For this review, take the finished solid that the model builds, in its own axes (mm). A direction names the side the tool comes from. Round coordinates to 2 decimals unless told otherwise and drop trailing zeros. Order: outer loops, then holes, each group sorted by start corner. A loop starts at its lowest first (then second) coordinate and runs counter-clockwise, first axis right, second up. Notation, with made-up numbers: (81, -17) -> (136, -17) arc R20 cw to (136, 10) -> close; hole circle Ø8 at (0, 13.25). An arc over 180 degrees is marked (long way). Use a Markdown table: item, result. Add a question column.
1) Machinability: for faces 4 (the face through (3, 54, -14)), 5 (the face through (-38.556, 93.156, -36.092)), 6 (the face through (-34.17, 64.54, -36.5)), 7 (the face through (-3, 54, -14)), which of the approach directions +Z, -Z, +X, -X, +Y, -Y give a long, thin tool a straight path to every point of the face, cutting with its end or side? Answer none if there is none.
2) Wall thickness on line 1 along Y through (x, z) = (-36, 27); line 2 along Y through (x, z) = (-32, 16.5); line 3 along Z through (x, y) = (17, 89.5): over which ranges is each line inside the solid? List them lowest first. Write a range as [from, to].
3) Consider section B-B (y = 23). State the section outline as (x, z) points.
4) Consider section A-A (y = 101.5). State the section outline as (x, z) points, plus the area to 3 significant figures.
5) Clearance check with flat-ended pins moving along their axes: P1, Ø3.5, axis at y = 54.5, z = -14, coming from the +X side; P2, Ø1.5, axis at y = 55.5, z = -11, coming from the -X side; P3, Ø12, axis at x = -7, z = -46.5, coming from the -Y side. State where each tip first meets the part, or that it passes through.
6) Consider section C-C (y = 9). State the section outline as (x, z) points.
7) Draft analysis for pull direction Y (two halves, no side actions). For faces 1 (the face through (-34, 109, -34)), 2 (the face through (-10, 0, -10)), 3 (the face through (-38.327, 95.965, -35.879)), state which applies: pulls with the +Y half, pulls with the -Y half, needs draft (parallel to the pull), parting line crosses it, or undercut.
Autodesk Fusion 360 part; units mm, degrees
sketch "Sketch1" plane through (0, 0, 0) normal (0, 0, 1) x (1, 0, 0)
  line L0 (12.5, 0) -> (22.5, 0)
  line L1 (12.5, 0) -> (12.5, 20)
  line L2 (22.5, 0) -> (22.5, 20)
  line L3 (22.5, 20) -> (42.5, 20)
  line L4 (42.5, 20) -> (42.5, 25)
  line L5 (42.5, 25) -> (22.5, 25)
  line L6 (0, 0) -> (0, 115)
  line L7 (0, 25) -> (0, 41)
  line L8 (22.5, 41) -> (47.5, 41)
  line L9 (47.5, 41) -> (47.5, 46)
  line L10 (47.5, 46) -> (22.5, 46)
  line L11 (0, 46) -> (0, 62)
  line L12 (22.5, 62) -> (50, 62)
  line L13 (50, 62) -> (50, 67)
  line L14 (50, 67) -> (22.5, 67)
  line L15 (0, 67) -> (0, 83)
  line L16 (57.5, 83) -> (57.5, 88)
  line L17 (0, 88) -> (0, 104)
  line L18 (65, 104) -> (65, 109)
  line L19 (52.5, 98.5) -> (52.5, 93.5)
  line L20 (65, 104) -> (52.5, 98.5)
  line L21 (52.5, 93.5) -> (57.5, 88)
  line L22 (12.5, 20) -> (12.5, 109)
  line L23 (22.5, 20) -> (22.5, 109)
  line L24 (0, 83) -> (0, 77.5)
  line L25 (23, 77.5) -> (42.5, 77.5)
  line L26 (42.5, 77.5) -> (42.5, 72.5)
  line L27 (42.5, 72.5) -> (22.5, 72.5041)
  line L28 (42.5, 77.5) -> (57.5, 83)
  line L29 (42.5, 72.5) -> (50, 67)
  line L30 (0, 62) -> (0, 56.5)
  line L31 (22.5, 56.5) -> (35, 56.5)
  line L32 (35, 56.5) -> (35, 51.5)
  line L33 (35, 56.5) -> (50, 62)
  line L34 (35, 51.5) -> (47.5, 46)
  line L35 (0, 41) -> (0, 35.5)
  line L36 (22.5, 35.5) -> (27.5, 35.5)
  line L37 (27.5, 35.5) -> (27.5, 30.5)
  line L38 (47.5, 41) -> (27.5, 35.5)
  line L39 (27.5, 30.5) -> (42.5, 25)
  line L40 (0, 93.5) -> (-0.0024, 93.5)
  line L41 (35, 51.5) -> (22.5, 51.5)
  line L42 (0, 51.5) -> (-0.0011, 51.5)
  line L43 (27.5, 30.5) -> (22.5, 30.5)
  line L44 (0, 30.5) -> (-0.1134, 30.5)
  line L45 (12.5, 109) -> (12.5, 64)
  line L46 (22.5, 76.8571) -> (47.5, 109)
  line L47 (43.6111, 104) -> (65, 104)
  line L48 (39.3333, 98.5) -> (52.5, 98.5)
  line L49 (52.5, 93.5) -> (35.4444, 93.5)
  line L50 (57.5, 88) -> (31.1667, 88)
  line L51 (27.2778, 83) -> (57.5, 83)
  line L52 (65, 109) -> (47.5, 109)
  line L53 (22.5, 109) -> (12.5, 109)
  line L54 (27.2778, 83) -> (22.5, 83)
  dimension "d1" = 12.5
  dimension "d2" = 22.5
  dimension "d3" = 20
  dimension "d6" = 5
  dimension "d7" = 115
  dimension "d8" = 16
  dimension "d9" = 47.5
  dimension "d10" = 5
  dimension "d11" = 16
  dimension "d12" = 50
  dimension "d13" = 5
  dimension "d14" = 16
  dimension "d15" = 57.5
  dimension "d16" = 5
  dimension "d17" = 16
  dimension "d18" = 65
  dimension "d19" = 5
  dimension "d24" = 5
  dimension "d25" = 90
  dimension "d26" = 5.5
  dimension "d27" = 42.5
  dimension "d28" = 5
  dimension "d29" = 5.5
  dimension "d30" = 35
  dimension "d31" = 5
  dimension "d32" = 90
  dimension "d33" = 5.5
  dimension "d34" = 27.5
  dimension "d35" = 5
  dimension "d36" = 90
  dimension "d37" = 45
  dimension "d38" = 25
revolve "Revolve1" add sketch "Sketch1" angle 360 about axis through (0, 0, 0) along (0, 1, 0)
sketch "Sketch2" plane through (0, 0, 0) normal (0, 1, 0) x (1, 0, 0)
  line L0 (0, 12.5) -> (0, 15.5)
  line L1 (0, 15.5) -> (3, 15.5)
  line L2 (3, 15.5) -> (-3, 15.5)
  line L3 (-3, 15.5) -> (-3, 12)
  line L4 (-3, 12) -> (3, 12)
  line L5 (3, 12) -> (3, 15.5)
  dimension "d40" = 3
  dimension "d41" = 6
extrude "Extrude1" cut sketch "Sketch2" along normal blind 115
sketch "Sketch3" plane through (0, 0, 0) normal (0, 1, 0) x (1, 0, 0)
  line L0 (0, -90) -> (100, -90)
  line L1 (100, -90) -> (100, 0)
  line L2 (100, 0) -> (0, 0)
  line L3 (0, 0) -> (0, -90)
extrude "Extrude2" cut sketch "Sketch3" along normal blind 115
Results list:
| question | item | result |
|---|---|---|
| 1 | face 4 | +Z, +Y, -Y |
| 1 | face 5 | none |
| 1 | face 6 | -Y |
| 1 | face 7 | +Y, -Y |
| 2 | line 1 | [40.31, 47.1], [60.17, 70.67], [78.42, 105.79] |
| 2 | line 2 | [20, 27.38], [37.84, 51.06], [56.87, 94.22] |
| 2 | line 3 | [-53.5, -27.5], [-14.74, 0] |
| 3 | outline | (-3, -15.5) -> (-3, -12.13) arc R12.5 cw to (0, 12.5) -> (0, 42.5) arc R42.5 ccw (long way) to (42.5, 0) -> (12.5, 0) arc R12.5 cw to (3, -12.13) -> (3, -15.5) -> close |
| 4 | outline | (-3, -15.5) -> (-3, -12.13) arc R12.5 cw to (0, 12.5) -> (0, 22.5) arc R22.5 ccw (long way) to (22.5, 0) -> (12.5, 0) arc R12.5 cw to (3, -12.13) -> (3, -15.5) -> close; (0, 41.67) -> (0, 59.32) arc R59.32 ccw (long way) to (59.32, 0) -> (41.67, 0) arc R41.67 cw (long way) to start |
| 4 | area | 5,010 mm2 |
| 5 | P1 | x = 32.79 |
| 5 | P2 | x = -33.47 |
| 5 | P3 | y = 20 |
| 6 | outline | (-3, -15.5) -> (-3, -12.13) arc R12.5 cw to (0, 12.5) -> (0, 22.5) arc R22.5 ccw (long way) to (22.5, 0) -> (12.5, 0) arc R12.5 cw to (3, -12.13) -> (3, -15.5) -> close |
| 7 | face 1 | pulls with the +Y half |
| 7 | face 2 | pulls with the -Y half |
| 7 | face 3 | undercut |
